The drawing under review shows one solid part. Ordinate dimensions are in mm from its lowest x, y, z. Coordinates: 2 decimals unless noted, no trailing zeros. Loops run counter-clockwise (first coordinate to the right, second up) from the corner with the lowest first, then second, coordinate; pieces in that order, holes last. Notation, with made-up numbers: M 84,51 L 137,51 A17 cw 137,77 Z; hole C 27,18.5 d4. An arc over 180 degrees is marked long. Return JSON: item names as keys, results as strings.
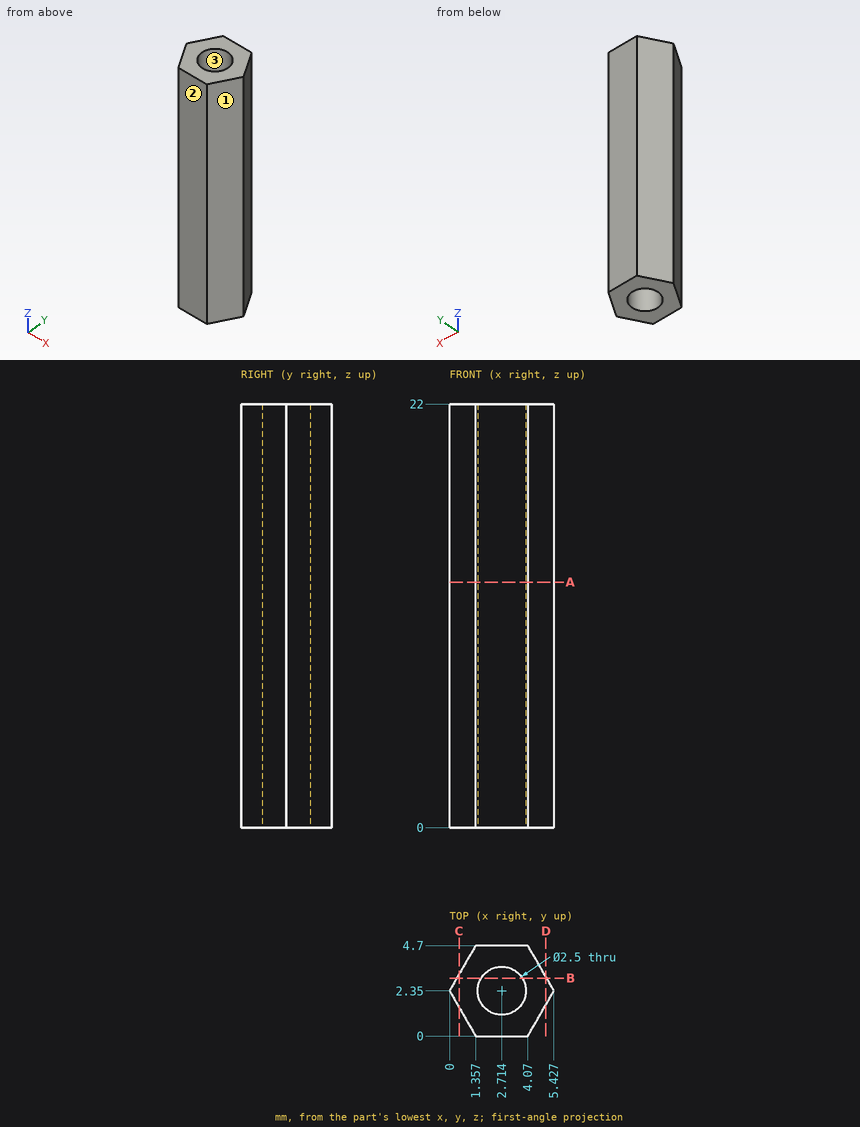
1. Add section C-C on x = 0.5. Give the boundary of the cut face in (y, z), plus the area to 3 significant figures.
Check values:
{"outline": "M 1.48,0 L 3.22,0 L 3.22,22 L 1.48,22 Z", "area": "38.1 mm²"}
2. The part is to be moulded in two halves that separate along X. For the marked faces 1, 2 and 3, say which applies: released by +X, released by -X, zero draft, split by the parting line, or undercut.
Check values:
{"face 1": "released by +X", "face 2": "zero draft", "face 3": "undercut"}
3. Add section D-D on x = 5. Give the boundary of the cut face in (y, z).
Check values:
{"outline": "M 1.61,0 L 3.09,0 L 3.09,22 L 1.61,22 Z"}
4. To check wall thickness, follow line 1 (Y direction, x = 2.8, z = 15.5); line 2 (Y direction, x = 3.75, z = 10.25); line 3 (X direction, y = 2.3, z = 8) (1 decimal). State the ranges of each line that lie inside material, in increasing order.
Check values:
{"line 1": "0 to 1.1, 3.6 to 4.7", "line 2": "0 to 1.65, 3.05 to 4.7", "line 3": "0 to 1.5, 4 to 5.4"}
5. Insertion check: pin 1 Ø1 at (x, z) = (4.5, 19.5) entering from -Y; pin 2 Ø1.5 at (y, z) = (4, 9.5) entering from +X. Each pin has a flat end and moves straight along its axis. Give the tip position at first contact, or say it passes through.
Check values:
{"pin 1": "y = 0", "pin 2": "x = 4.91"}
6. Add section A-A on z = 12.75. Give the boundary of the cut face in (x, y), plus the area to 3 significant figures.
Check values:
{"outline": "M 0,2.35 L 1.36,0 L 4.07,0 L 5.43,2.35 L 4.07,4.7 L 1.36,4.7 Z; hole C 2.71,2.35 d2.5", "area": "14.2 mm²"}
7. Add section B-B on y = 3. Give the boundary of the cut face in (x, z) (1 decimal).
Check values:
{"outline": "M 0.4,0 L 1.6,0 L 1.6,22 L 0.4,22 Z; M 3.8,0 L 5.1,0 L 5.1,22 L 3.8,22 Z"}
